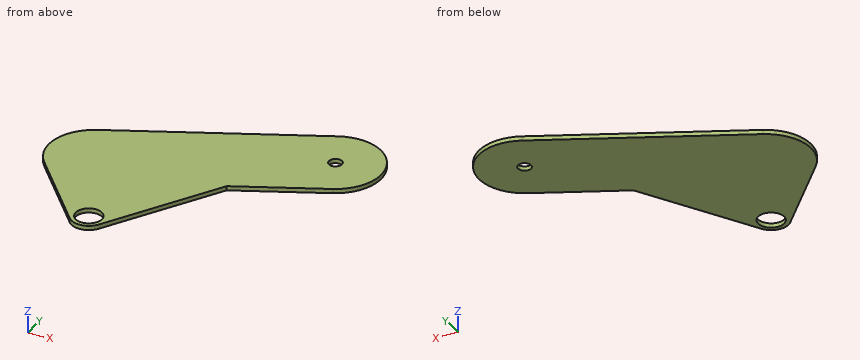
Autodesk Inventor part; units mm, degrees
ref_plane "YZ Plane" through (0, 0, 0) normal (1, 0, 0) x (0, 1, 0)
ref_plane "XZ Plane" through (0, 0, 0) normal (0, 1, 0) x (-1, 0, 0)
ref_plane "XY Plane" through (0, 0, 0) normal (0, 0, 1) x (1, 0, 0)
sketch "スケッチ1" plane through (0, 0, 0) normal (0, 0, 1) x (1, 0, 0)
  circle A0 centre (23.2, 20.8573) radius 3
  circle A1 centre (56.5578, 64) radius 1.5
  line L0 (23.2, 20.8573) -> (56.5578, 64)
  line L1 (23.2, 20.8573) -> (56.5578, 64) construction
  circle A2 centre (56.5578, 64) radius 1.5
  line L2 (23.2, 20.8573) -> (12.5297, 42.1181)
  line L3 (12.5297, 42.1181) -> (56.5578, 64) construction
  line L4 (17.2029, 32.7153) -> (61.231, 54.5973)
  line L5 (51.8846, 73.4027) -> (7.8565, 51.5208)
  arc A3 (7.8565, 51.5208) -> (17.2029, 32.7153) centre (12.5297, 42.1181) ccw
  arc A4 (61.231, 54.5973) -> (51.8846, 73.4027) centre (56.5578, 64) ccw
  circle A5 centre (23.2, 20.8573) radius 4
  line L6 (4.7893, 35.0232) -> (20.2513, 18.1545)
  line L7 (41.8337, 44.9568) -> (26.6583, 18.8472)
  point P0 (0, 0)
  point P1 (0, 0)
  point P2 (39.8789, 42.4286)
  point P3 (34.5437, 53.059)
  point P4 (26.2844, 23.4042)
  point P5 (20.1698, 18.2461)
  point P6 (25.5392, 22.7356)
  point P7 (21.8543, 23.5385)
  point P8 (21.4058, 24.4323)
  point P9 (25.6467, 24.0217)
  point P10 (25.035, 23.2306)
  dimension "d6" = 3
  dimension "d7" = 21
  dimension "d8" = 8
extrude "押し出し1" add sketch "スケッチ1" along normal blind 1 contours A0 L0 A5 L2 | A0 L2 A5 L0 | A5 L2 L4 L0 | L0 L7 A5 | A5 L6 A3 L4 L2 | L4 A3 L5 A4
properties part number "ダンパーガード" material "ポリカーボネート、クリア"
Check sheet for the modelled part. Datum: model origin and axes. Units: mm. Coordinates: 2 decimals unless noted, no trailing zeros. Loops run counter-clockwise (first coordinate to the right, second up) from the corner with the lowest first, then second, coordinate; pieces in that order, holes last. Notation, with made-up numbers: (16, 71.25) -> (71, 71.25) arc R31 cw to (71, 103.25) -> close; hole circle Ø9 at (-14, -36). An arc over 180 degrees is marked (long way). Write item = value, one per line. Start each with the question number.
1. Material ranges on line 1 (Y direction, x = 23.2, z = 0.6); line 2 (X direction, y = 64, z = 0.45); line 3 (X direction, y = 21.5, z = 0.7), recorded low to high.
2. Section check C-C on z = 0.25. Record the cut outline in (x, y).
3. Depth check by flat-ended pin: P1, Ø2.5, axis at x = 56.56, y = 64, coming from the -Z side; P2, Ø6, axis at x = 19, y = 43.5, coming from the -Z side. Enter the tip coordinate at first touch or a pass-through.
4. Section check B-B on x = 23.2. Record the cut outline in (y, z).
5. Section check D-D on y = 58. Record the cut outline in (x, z), then the cut area to 3 significant figures.
6. Section check A-A on y = 64. Record the cut outline in (x, z).
Responses:
q1.line_1 = 16.86 to 17.86, 23.86 to 59.15
q1.line_2 = 32.97 to 55.06, 58.06 to 67.06
q1.line_3 = 17.18 to 20.27, 26.13 to 28.2
q2.outline = (4.79, 35.02) -> (20.25, 18.15) arc R4 ccw to (26.66, 18.85) -> (41.83, 44.96) -> (61.23, 54.6) arc R10.5 ccw to (51.88, 73.4) -> (7.86, 51.52) arc R10.5 ccw to start; hole circle Ø6 at (23.2, 20.86); hole circle Ø3 at (56.56, 64)
q3.P1 = through
q3.P2 = 0
q4.outline = (16.86, 0) -> (17.86, 0) -> (17.86, 1) -> (16.86, 1) -> close; (23.86, 0) -> (59.15, 0) -> (59.15, 1) -> (23.86, 1) -> close
q5.outline = (20.89, 0) -> (65.17, 0) -> (65.17, 1) -> (20.89, 1) -> close
q5.area = 44.3 mm2
q6.outline = (32.97, 0) -> (55.06, 0) -> (55.06, 1) -> (32.97, 1) -> close; (58.06, 0) -> (67.06, 0) -> (67.06, 1) -> (58.06, 1) -> close
